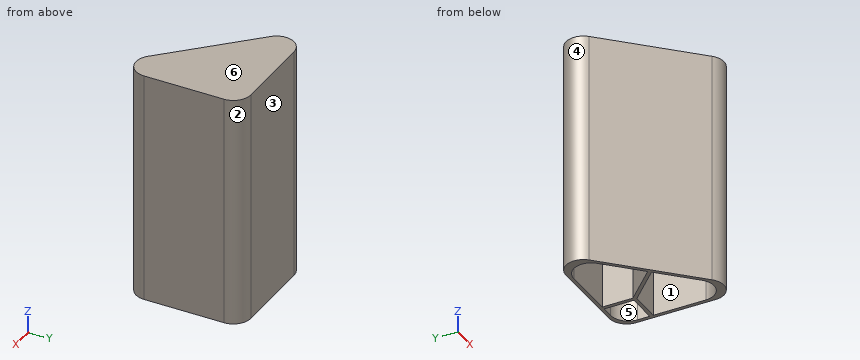
```python
from build123d import *

# Parameters (mm, degrees)
F0_W      = 17
F0_H      = 17
F1_DEPTH  = 100
F4_DEPTH  = 2
F7_DEPTH  = 30
F10_DEPTH = 2
F11_R     = 10


with BuildPart() as f1:
    # F0 (on Top) → F1 (new body)
    with BuildSketch(Plane.XY):
        Polygon((40, -37.3566303961), (40, 40), (-40, 40), (-38, 38), (40, -40), align=None)
        Polygon((20.4142135624, 19), (38, 19), (38, -35.3566303961), (2.0287915831, 0.6145780208), align=None, mode=Mode.SUBTRACT)
        Polygon((19, 20.4142135624), (0.6145780208, 2.0287915831), (-35.3566303961, 38), (19, 38), align=None, mode=Mode.SUBTRACT)
        with Locations((29.5, 29.5)):
            Rectangle(F0_W, F0_H, mode=Mode.SUBTRACT)
    extrude(amount=F1_DEPTH)

    # F3 (on offset) → F4 (join)
    with BuildSketch(Plane.XY.offset(100)):
        Polygon((40, 40), (-40, 40), (0, 0), (40, -40), align=None)
        Polygon((21.0052309155, 18.2000048862), (37.2052026456, 18.2302694688), (37.3013024139, -33.2098427904), (3.2906330243, 0.673986953), (20.7508157718, 18.199529591), align=None, mode=Mode.SUBTRACT)
        Polygon((0.7071067812, 3.2526911935), (-33.2402020254, 37.2), (18.2, 37.2), (18.2, 21), (18.2, 20.7455844123), align=None, mode=Mode.SUBTRACT)
        Polygon((37.999970334, 21.03175913), (21, 21), (21, 38), (37.9682704806, 38), align=None, mode=Mode.SUBTRACT)
    extrude(amount=F4_DEPTH)

    # F6 (on offset) → F7 (join)
    with BuildSketch(Plane.XY.offset(102)):
        Polygon((40, -40), (40, 40), (-40, 40), align=None)
        Polygon((-35.1715728753, 38), (38, 38), (38, -35.1715728753), align=None, mode=Mode.SUBTRACT)
    extrude(amount=F7_DEPTH)

    # F9 (on offset) → F10 (join)
    with BuildSketch(Plane.XY.offset(132)):
        Polygon((40, -40), (40, 40), (-40, 40), align=None)
    extrude(amount=F10_DEPTH)

    # F11
    f11_edges = [f1.edges().sort_by_distance(p)[0] for p in [
        (-35.35663, 38, 50),
        (-33.240202, 37.2, 101),
        (-35.171573, 38, 117),
        (-40, 40, 67),
        (38, -35.35663, 50),
        (40, -40, 67),
        (37.301302, -33.209843, 101),
        (38, -35.171573, 117),
        (38, 38, 50),
        (40, 40, 67),
    ]]
    fillet(f11_edges, radius=F11_R)


solid = f1.part
```
Could you check a few things on this model? Use its own coordinates, in mm. Face numbers are marked on the shaded views. A direction names the side the tool comes from. Round coordinates to 2 decimals unless told otherwise and drop trailing zeros. Loops run counter-clockwise (first coordinate to the right, second up) from the corner with the lowest first, then second, coordinate; pieces in that order, holes last. Notation, with made-up numbers: (35, 38) - (92, 38) arc R15 cw to (92, 51) - close; hole circle Ø7 at (18, -29.75). An arc over 180 degrees is marked (long way). Answer in a Markdown table with one row per item. Add a question column.
(1) If we mould it in two halves opening along Y, with no side actions, what happens to the marked faces 3, 4, 5 and 6? For each: pulls with the +Y half, pulls with the -Y half, needs draft (parallel to the pull), parting line crosses it, or undercut.
(2) I need wall thicknesses on line 1 along X through (y, z) = (36, 53.5); line 2 along X through (y, z) = (25.5, 59.5); line 3 along Y through (x, z) = (23, 11). Which ranges of each line are inside material? Lowest first, please.
(3) If we section it at A-A (z = 24): Please give me the cut outline in (x, y), plus the area to 3 significant figures.
(4) If we section it at B-B (x = 7.5): Please give me the cut outline in (y, z).
(5) For the marked faces 1 and 2, which set-ups out of +Z, -Z, +X, -X, +Y, -Y let a thin tool reach every point of the face, with its end or its side?
(6) I'm going to push flat-ended pins straight in: pin 1 (2 mm diameter, centred on x = -2, z = 100.5, fed in from -Y); pin 2 (1.6 mm diameter, centred on y = 29, z = 100.5, fed in from -X); pin 3 (2 mm diameter, centred on y = -0.5, z = 18.5, fed in from -X). Where does each tip first touch, or does it pass through?
(7) If we section it at D-D (z = 126.5): Please give me the cut outline in (x, y).
Model answer:
| question | item | result |
|---|---|---|
| 1 | face 3 | pulls with the +Y half |
| 1 | face 4 | parting line crosses it |
| 1 | face 5 | undercut |
| 1 | face 6 | needs draft |
| 2 | line 1 | x = -23.86 to -17.21, 19 to 21, 34 to 38 |
| 2 | line 2 | x = -24.79 to -20.9, 19 to 21, 38 to 40 |
| 2 | line 3 | y = -23 to -19.87, 19 to 21, 38 to 40 |
| 3 | outline | (-22.93, 22.93) - (22.93, -22.93) arc R10 ccw to (40, -15.86) - (40, 30) arc R10 ccw to (30, 40) - (-15.86, 40) arc R10 ccw to start; hole (-18.29, 20.93) - (0.61, 2.03) - (19, 20.41) - (19, 38) - (-11.21, 38) arc R10 ccw to start; hole (2.03, 0.61) - (20.93, -18.29) arc R10 ccw to (38, -11.21) - (38, 19) - (20.41, 19) - close; hole (21, 21) - (38, 21) - (38, 28) arc R10 ccw to (28, 38) - (21, 38) - close |
| 3 | area | 632 mm² |
| 4 | outline | (-7.5, 0) - (-4.86, 0) - (-4.86, 100) - (-3.52, 100) - (-3.52, 102) - (-4.67, 102) - (-4.67, 132) - (38, 132) - (38, 102) - (37.2, 102) - (37.2, 100) - (38, 100) - (38, 0) - (40, 0) - (40, 134) - (-7.5, 134) - close; (4.9, 100) - (6.09, 100) - (6.09, 0) - (8.91, 0) - (8.91, 100) - (10.05, 100) - (10.05, 102) - (4.9, 102) - close |
| 5 | face 1 | -Z |
| 5 | face 2 | +Z, -Z, +X, +Y |
| 6 | pin 1 | stops at y = 1 |
| 6 | pin 2 | stops at x = -25.86 |
| 6 | pin 3 | stops at x = -0.5 |
| 7 | outline | (-22.93, 22.93) - (22.93, -22.93) arc R10 ccw to (40, -15.86) - (40, 30) arc R10 ccw to (30, 40) - (-15.86, 40) arc R10 ccw to start; hole (-18.1, 20.93) - (20.93, -18.1) arc R10 ccw to (38, -11.03) - (38, 28) arc R10 ccw to (28, 38) - (-11.03, 38) arc R10 ccw to start |
